Here's how the part is built. I have some questions about the finished solid (model axes, mm). Face numbers are marked on the shaded views. Coordinates: 2 decimals unless noted, no trailing zeros. Write each loop counter-clockwise with the first axis right and the second up, starting at its lowest first coordinate (ties: lowest second). Pieces come first, ordered by that corner, then holes. Notation, with made-up numbers: (68, -28.75) - (89, -28.75) arc R28 ccw to (89, 6.25) - close; hole circle Ø8 at (3.25, 3.5). An arc over 180 degrees is marked (long way). Answer in a Markdown table with one row per item. Add a question column.
Item 1: Imagine slicing it at B-B (z = 10.5). Please give me the cut outline in (x, y).
Item 2: We'd pull the mould along X, two halves only. Please class the marked faces 1, 2 and 3: +X half, -X half, draft (parallel to the pull), parting line (faces both ways), or undercut.
Item 3: Imagine slicing it at C-C (y = 1.75). Please give me the cut outline in (x, z).
Item 4: Imagine slicing it at A-A (x = 0). Please give me the cut outline in (y, z), plus the area to 3 significant figures.
Item 5: I'm going to push flat-ended pins straight in: pin 1 (1 mm diameter, centred on x = 14.5, y = -9.5, fed in from +Z); pin 2 (8 mm diameter, centred on x = -5.5, y = 0.5, fed in from +Z); pin 3 (2 mm diameter, centred on y = -0.5, z = 11.5, fed in from +X). Where does each tip first touch, or does it pass through?
Item 6: Imagine slicing it at D-D (y = -9). Please give me the cut outline in (x, z).
Item 7: If I drill on probe 1 along Z at (x, y) = (0, -4.75); probe 2 along Z at (x, y) = (7.5, -3.75); probe 3 along Z at (x, y) = (0, -9), over which ranges is the centre line in solid material (lowest first)? Write a range as from..to.
from build123d import *

# Parameters (mm, degrees)
F1_DEPTH = 16
F2_DEPTH = 3
F4_DEPTH = 8


with BuildPart() as f1:
    # F0 (on Front) → F1 (new body)
    with BuildSketch(Plane.XZ):
        with BuildLine():
            Line((15.5, 0), (13.5, 0))
            ThreePointArc((13.5, 0), (0, -13.5), (-13.5, 0))
            Line((-13.5, 0), (-15.5, 0))
            ThreePointArc((-15.5, 0), (0, -15.5), (15.5, 0))
        make_face()
    extrude(amount=F1_DEPTH)

    # F0 (on Front) → F2 (join)
    with BuildSketch(Plane.XZ):
        with BuildLine():
            Line((15.5, 0), (13.5, 0))
            ThreePointArc((13.5, 0), (0, -13.5), (-13.5, 0))
            Line((-13.5, 0), (-15.5, 0))
            ThreePointArc((-15.5, 0), (0, -15.5), (15.5, 0))
        make_face()
        with BuildLine():
            ThreePointArc((-13.5, 0), (0, -13.5), (13.5, 0))
            ThreePointArc((13.5, 0), (0, 13.5), (-13.5, 0))
        make_face()
    extrude(amount=-F2_DEPTH)

    # F3 (on face) → F4 (join)
    with BuildSketch(Plane(origin=(0, 3, 0), x_dir=(-1, 0, 0), z_dir=(0, 1, 0))):
        with BuildLine():
            Line((13.5, 0), (15.5, 0))
            ThreePointArc((15.5, 0), (0, 15.5), (-15.5, 0))
            Line((-15.5, 0), (-13.5, 0))
            ThreePointArc((-13.5, 0), (0, 13.5), (13.5, 0))
        make_face()
    extrude(amount=-F4_DEPTH)


solid = f1.part
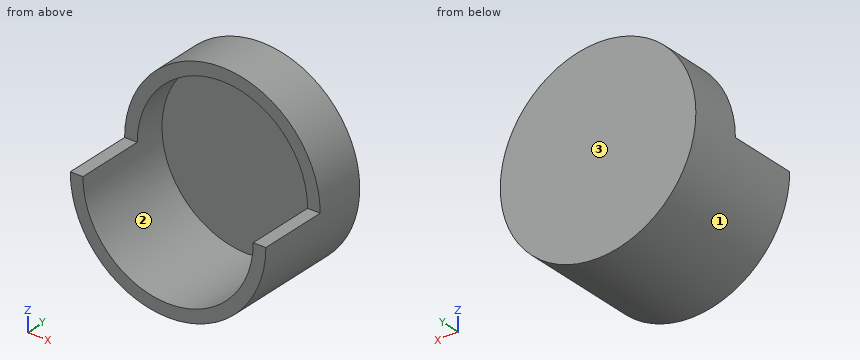
Here are the results:
| question | item | result |
|---|---|---|
| 1 | outline | (-11.4, -5) - (-8.49, -5) - (-8.49, 0) - (8.49, 0) - (8.49, -5) - (11.4, -5) - (11.4, 3) - (-11.4, 3) - close |
| 2 | face 1 | parting line |
| 2 | face 2 | undercut |
| 2 | face 3 | draft |
| 3 | outline | circle Ø31 at (0, 0) |
| 4 | outline | (-16, -15.5) - (3, -15.5) - (3, 15.5) - (-5, 15.5) - (-5, 13.5) - (0, 13.5) - (0, -13.5) - (-16, -13.5) - close |
| 4 | area | 135 mm2 |
| 5 | pin 1 | stops at z = 0 |
| 5 | pin 2 | stops at z = 15.43 |
| 5 | pin 3 | stops at x = 11.4 |
| 6 | outline | (-15.5, 0) arc R15.5 ccw to (15.5, 0) - (13.5, 0) arc R13.5 cw to (-13.5, 0) - close |
| 7 | probe 1 | z = -15.5..-13.5, 13.5..15.5 |
| 7 | probe 2 | z = -13.56..-11.22, 11.22..13.56 |
| 7 | probe 3 | z = -15.5..-13.5 |
